Verification items for the finished model (mm, model axes). Round coordinates to 2 decimals unless told otherwise and drop trailing zeros. Write each loop counter-clockwise with the first axis right and the second up, starting at its lowest first coordinate (ties: lowest second). Pieces come first, ordered by that corner, then holes. Notation, with made-up numbers: M 67.25,42 L 93.25,42 A13 cw 93.25,60 Z; hole C 86,25.5 d4. An arc over 180 degrees is marked long. One line per question, with ' | ' between items. Start each with the question number.
Q1. Cross-section at C-C (y = 14). Record the boundary of the cut face in (x, z), then the cut area to 3 significant figures.
Q2. Gauge pin test, flat ends, axial feed: pin 1 (1.5 mm diameter, centred on y = 31, z = 1, fed in from +X); pin 2 (1 mm diameter, centred on y = 12.5, z = 0, fed in from +X). Record the tip position at first contact, or that the pin passes through.
Q3. Thickness scan on line 1 along X through (y, z) = (0.5, -0.8); line 2 along Y through (x, z) = (23, 0); line 3 along X through (y, z) = (-43, -1.25). Record the ranges inside material, lowest first. Write a range as from..to.
Q4. Cross-section at B-B (z = -0.9). Record the boundary of the cut face in (x, y), then the cut area to 3 significant figures.
Q5. Cross-section at A-A (x = 0). Record the boundary of the cut face in (y, z), then the cut area to 3 significant figures.
from build123d import *

# Parameters (mm, degrees)
F0_R     = 55
F1_DEPTH = 1.5


with BuildPart() as f1:
    # F0 (on Top) → F1 (new body, symmetric)
    with BuildSketch(Plane.XY):
        Circle(F0_R)
        with BuildLine():
            ThreePointArc((-48.572008, -18), (-50.986616, -9.143576), (-51.8, 0))
            ThreePointArc((-51.8, 0), (-50.986616, 9.143576), (-48.572008, 18))
            ThreePointArc((-48.572008, 18), (0, 51.8), (48.572008, 18))
            ThreePointArc((48.572008, 18), (50.986616, 9.143576), (51.8, 0))
            ThreePointArc((51.8, 0), (50.986616, -9.143576), (48.572008, -18))
            ThreePointArc((48.572008, -18), (0, -51.8), (-48.572008, -18))
        make_face(mode=Mode.SUBTRACT)
    extrude(amount=F1_DEPTH, both=True)


solid = f1.part
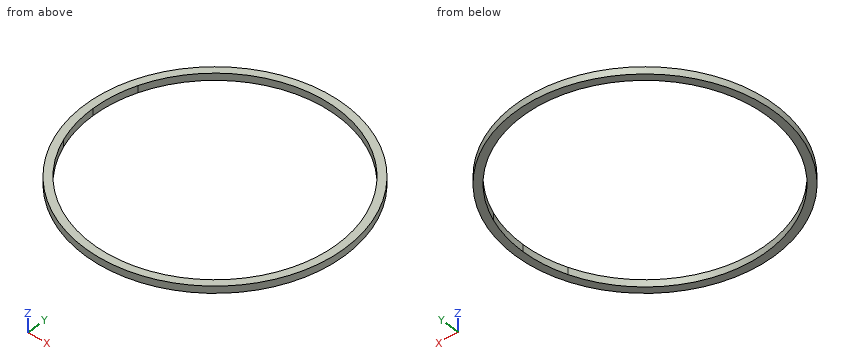
Determined:
1) outline: M -53.19,-1.5 L -49.87,-1.5 L -49.87,1.5 L -53.19,1.5 Z; M 49.87,-1.5 L 53.19,-1.5 L 53.19,1.5 L 49.87,1.5 Z | area: 19.9 mm²
2) pin 1: stops at x = 45.93 | pin 2: stops at x = 53.67
3) line 1: x = -55..-51.8, 51.8..55 | line 2: y = -49.96..-46.41, 46.41..49.96 | line 3: x = -34.29..-28.88, 28.88..34.29
4) outline: C 0,0 d110; hole M -48.57,-18 A51.8 ccw 48.57,-18 A51.8 ccw 48.57,18 A51.8 ccw -48.57,18 A51.8 ccw Z | area: 1,070 mm²
5) outline: M -55,-1.5 L -51.8,-1.5 L -51.8,1.5 L -55,1.5 Z; M 51.8,-1.5 L 55,-1.5 L 55,1.5 L 51.8,1.5 Z | area: 19.2 mm²
